from build123d import *

# Parameters (mm, degrees)
SKETCH1_R           = 26.67
BOSS_EXTRUDE1_DEPTH = 3.175
CUT_EXTRUDE1_REACH  = 144.628
CUT_EXTRUDE2_REACH  = 144.628
SKETCH3_R           = 2.665
FILLET1_R           = 2.54


with BuildPart() as part:
    # Sketch1 → Boss-Extrude1 (new body)
    with BuildSketch(Plane.XY):
        with BuildLine():
            Line((-34.925, 0), (-34.925, -63.5))
            Line((-34.925, -63.5), (-34.925, -103.175))
            Line((-34.925, -103.175), (98.425, -103.175))
            Line((98.425, -103.175), (98.425, -64.833888838))
            Line((98.425, -64.833888838), (98.425, 0))
            ThreePointArc((98.425, 0), (31.75, 66.675), (-34.925, 0))
        make_face()
        Circle(SKETCH1_R, mode=Mode.SUBTRACT)
    extrude(amount=BOSS_EXTRUDE1_DEPTH)

    # Sketch2 → Cut-Extrude1 (cut, up to next)
    with BuildSketch(Plane.XY.offset(3.175), mode=Mode.PRIVATE) as cut_extrude1_sk1:
        with BuildLine():
            Line((31.75, -66.675), (31.75, -103.175))
            Line((31.75, -103.175), (98.425, -103.175))
            Line((98.425, -103.175), (98.425, 0))
            ThreePointArc((98.425, 0), (78.896344636, -47.146344636), (31.75, -66.675))
        make_face()
    cut_extrude1_tool1 = extrude(cut_extrude1_sk1.sketch, amount=-CUT_EXTRUDE1_REACH, mode=Mode.PRIVATE) & part.part
    add(cut_extrude1_tool1.solids().sort_by_distance((70.281775, -75.59134, 3.175))[0], mode=Mode.SUBTRACT)

    # Sketch3 → Cut-Extrude2 (cut, up to next)
    with BuildSketch(Plane(origin=(0, 0, 0), x_dir=(-1, 0, 0), z_dir=(0, 0, -1)), mode=Mode.PRIVATE) as cut_extrude2_sk1:
        with Locations((-21.75, -93.175)):
            Circle(SKETCH3_R)
    cut_extrude2_tool1 = extrude(cut_extrude2_sk1.sketch, amount=-CUT_EXTRUDE2_REACH, mode=Mode.PRIVATE) & part.part
    # Sketch3 → Cut-Extrude2 (cut, up to next)
    with BuildSketch(Plane(origin=(0, 0, 0), x_dir=(-1, 0, 0), z_dir=(0, 0, -1)), mode=Mode.PRIVATE) as cut_extrude2_sk2:
        with Locations(Location((-21.75, -73.175, 0), (0, 0, 180))):
            Circle(SKETCH3_R)
    cut_extrude2_tool2 = extrude(cut_extrude2_sk2.sketch, amount=-CUT_EXTRUDE2_REACH, mode=Mode.PRIVATE) & part.part
    # Sketch3 → Cut-Extrude2 (cut, up to next)
    with BuildSketch(Plane(origin=(0, 0, 0), x_dir=(-1, 0, 0), z_dir=(0, 0, -1)), mode=Mode.PRIVATE) as cut_extrude2_sk3:
        with Locations(Location((24.925, -93.175, 0), (0, 0, 180))):
            Circle(SKETCH3_R)
    cut_extrude2_tool3 = extrude(cut_extrude2_sk3.sketch, amount=-CUT_EXTRUDE2_REACH, mode=Mode.PRIVATE) & part.part
    # Sketch3 → Cut-Extrude2 (cut, up to next)
    with BuildSketch(Plane(origin=(0, 0, 0), x_dir=(-1, 0, 0), z_dir=(0, 0, -1)), mode=Mode.PRIVATE) as cut_extrude2_sk4:
        with Locations((24.925, -73.175)):
            Circle(SKETCH3_R)
    cut_extrude2_tool4 = extrude(cut_extrude2_sk4.sketch, amount=-CUT_EXTRUDE2_REACH, mode=Mode.PRIVATE) & part.part
    add(cut_extrude2_tool1.solids().sort_by_distance((21.75, -93.175, 0))[0], mode=Mode.SUBTRACT)
    add(cut_extrude2_tool2.solids().sort_by_distance((21.75, -73.175, 0))[0], mode=Mode.SUBTRACT)
    add(cut_extrude2_tool3.solids().sort_by_distance((-24.925, -93.175, 0))[0], mode=Mode.SUBTRACT)
    add(cut_extrude2_tool4.solids().sort_by_distance((-24.925, -73.175, 0))[0], mode=Mode.SUBTRACT)

    # Fillet1
    fillet1_edges = [part.edges().sort_by_distance(p)[0] for p in [
        (-34.925, -103.175, 1.5875),
        (31.75, -66.675, 1.5875),
        (31.75, -103.175, 1.5875),
    ]]
    fillet(fillet1_edges, radius=FILLET1_R)


solid = part.part
Verification items for the finished model (mm, model axes). Give positions to 0.01 mm unless a question says otherwise; leave off trailing zeros. Write each loop counter-clockwise with the first axis right and the second up, starting at its lowest first coordinate (ties: lowest second). Pieces come first, ordered by that corner, then holes. Notation, with made-up numbers: (-6, 61.5) - (2, 61.5) arc R15 ccw to (2, 77.5) - close; hole circle Ø11 at (15, 36.25). An arc over 180 degrees is marked (long way). Answer as CSV lines item,"result". Start each with the question number.
1. Draft check along Y on faces 1 (the face through (-3.472, 26.443, 1.565)), 2 (the face through (31, -17, 3.175)). Enter one of: pulls with the +Y half, pulls with the -Y half, needs draft (parallel to the pull), parting line crosses it, or undercut.
2. Sectioned sample at C-C (x = 0). Record the boundary of the cut face in (y, z) (3 decimals), then the cut area to 3 significant figures.
3. Depth check by flat-ended pin: pin 1 (1.5 mm diameter, centred on x = 68, y = 29, fed in from -Z). Enter the tip coordinate at first touch or a pass-through.
4. Thickness scan on line 1 (X direction, y = -73, z = 1.15) (3 decimals); line 2 (Y direction, x = 22, z = 1.5) (3 decimals); line 3 (Y direction, x = 21.75, z = 2.35) (3 decimals). Record the ranges inside material, lowest first.
5. Sectioned sample at B-B (y = -7). Record the boundary of the cut face in (x, z) (3 decimals).
6. Sectioned sample at A-A (x = 22.5). Record the boundary of the cut face in (y, z) (3 decimals).
7. Sectioned sample at D-D (z = 1.15). Record the boundary of the cut face in (x, y) (3 decimals).
Derived:
1,face 1,"undercut"
1,face 2,"needs draft"
2,outline,"(-103.175, 0) - (-26.67, 0) - (-26.67, 3.175) - (-103.175, 3.175) - close; (26.67, 0) - (58.63, 0) - (58.63, 3.175) - (26.67, 3.175) - close"
2,area,"344 mm²"
3,pin 1,"z = 0"
4,line 1,"-34.925 to -27.584, -22.266 to 19.091, 24.409 to 31.75"
4,line 2,"-103.175 to -95.828, -90.522 to -75.828, -70.522 to -15.076, 15.076 to 65.958"
4,line 3,"-103.175 to -95.84, -90.51 to -75.84, -70.51 to -15.435, 15.435 to 65.921"
5,outline,"(-34.925, 0) - (-25.735, 0) - (-25.735, 3.175) - (-34.925, 3.175) - close; (25.735, 0) - (98.057, 0) - (98.057, 3.175) - (25.735, 3.175) - close"
6,outline,"(-103.175, 0) - (-95.732, 0) - (-95.732, 3.175) - (-103.175, 3.175) - close; (-90.618, 0) - (-75.732, 0) - (-75.732, 3.175) - (-90.618, 3.175) - close; (-70.618, 0) - (-14.319, 0) - (-14.319, 3.175) - (-70.618, 3.175) - close; (14.319, 0) - (66.03, 0) - (66.03, 3.175) - (14.319, 3.175) - close"
7,outline,"(-34.925, -100.635) arc R2.54 ccw to (-32.385, -103.175) - (29.21, -103.175) arc R2.54 ccw to (31.75, -100.635) - (31.75, -69.168) arc R2.54 cw to (34.197, -66.63) arc R66.675 ccw (long way) to (-34.925, 0) - close; hole circle Ø5.33 at (-24.925, -93.175); hole circle Ø5.33 at (-24.925, -73.175); hole circle Ø53.34 at (0, 0); hole circle Ø5.33 at (21.75, -93.175); hole circle Ø5.33 at (21.75, -73.175)"
